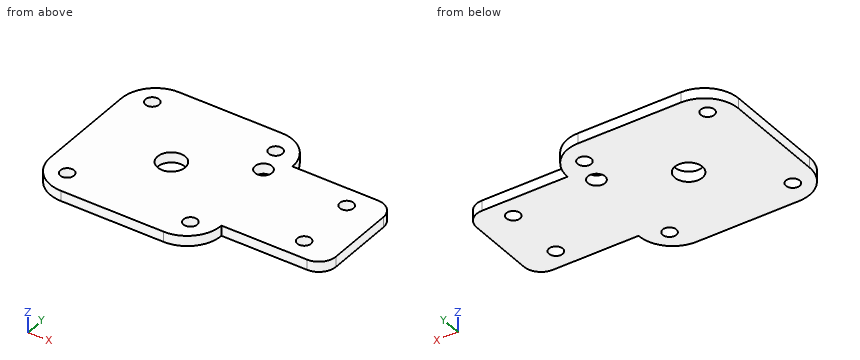
```python
from build123d import *

# Parameters (mm, degrees)
CROQUIS1_R              = 2.5
CROQUIS1_R_2            = 4.05
CROQUIS1_R_3            = 2
SALIENTE_EXTRUIR1_DEPTH = 3


with BuildPart() as part:
    # Croquis1 → Saliente-Extruir1 (new body)
    with BuildSketch(Plane.XY):
        with BuildLine():
            ThreePointArc((0, 40), (2.928932188, 47.071067812), (10, 50))
            Line((10, 50), (40, 50))
            ThreePointArc((40, 50), (47.071067812, 47.071067812), (50, 40))
            Line((50, 40), (50, 10))
            ThreePointArc((50, 10), (47.071067812, 2.928932188), (40, 0))
            Line((40, 0), (10, 0))
            ThreePointArc((10, 0), (2.928932188, 2.928932188), (0, 10))
            Line((0, 10), (0, 40))
        make_face()
        with Locations((45, 35)):
            Circle(CROQUIS1_R, mode=Mode.SUBTRACT)
        with Locations((25, 25)):
            Circle(CROQUIS1_R_2, mode=Mode.SUBTRACT)
        with Locations((43, 43)):
            Circle(CROQUIS1_R_3, mode=Mode.SUBTRACT)
        with Locations((7, 43)):
            Circle(CROQUIS1_R_3, mode=Mode.SUBTRACT)
        with Locations((43, 7)):
            Circle(CROQUIS1_R_3, mode=Mode.SUBTRACT)
        with Locations((7, 7)):
            Circle(CROQUIS1_R_3, mode=Mode.SUBTRACT)
        with BuildLine():
            ThreePointArc((75, 40), (78.535533906, 38.535533906), (80, 35))
            Line((80, 35), (80, 15))
            ThreePointArc((80, 15), (78.535533906, 11.464466094), (75, 10))
            Line((75, 10), (50, 10))
            Line((50, 10), (50, 40))
            Line((50, 40), (75, 40))
        make_face()
        with Locations((70, 16)):
            Circle(CROQUIS1_R_3, mode=Mode.SUBTRACT)
        with Locations((70, 34)):
            Circle(CROQUIS1_R_3, mode=Mode.SUBTRACT)
    extrude(amount=SALIENTE_EXTRUIR1_DEPTH)


solid = part.part
```
Check sheet for the modelled part. Datum: model origin and axes. Units: mm. Round coordinates to 2 decimals unless told otherwise and drop trailing zeros. Order: outer loops, then holes, each group sorted by start corner. A loop starts at its lowest first (then second) coordinate and runs counter-clockwise, first axis right, second up. Notation, with made-up numbers: M 34.5,-18 L 88.5,-18 A30 cw 88.5,9 Z; hole C 84.25,5.25 d8. An arc over 180 degrees is marked long. Answer in a Markdown table with one row per item.
(1) Section check A-A on x = 25. Record the boundary of the cut face in (y, z).
Findings:
| item | result |
|---|---|
| outline | M 0,0 L 20.95,0 L 20.95,3 L 0,3 Z; M 29.05,0 L 50,0 L 50,3 L 29.05,3 Z |
(2) Material ranges on line 1 along Y through (x, z) = (43, 2.35); line 2 along Y through (x, z) = (52.5, 2.55); line 3 along Y through (x, z) = (7, 1.85), recorded low to high. Write a range as from..to.
Findings:
| item | result |
|---|---|
| line 1 | y = 0.46..5, 9..33.5, 36.5..41, 45..49.54 |
| line 2 | y = 10..40 |
| line 3 | y = 0.46..5, 9..41, 45..49.54 |
(3) Gauge pin test, flat ends, axial feed: pin 1 (2.5 mm diameter, centred on x = 70, y = 16, fed in from -Z); pin 2 (0.9 mm diameter, centred on x = 58.5, z = 1.5, fed in from -Y). Record the tip position at first contact, or that the pin passes through.
Findings:
| item | result |
|---|---|
| pin 1 | passes through |
| pin 2 | stops at y = 10 |
(4) Section check C-C on y = 43. Record the boundary of the cut face in (x, z).
Findings:
| item | result |
|---|---|
| outline | M 0.46,0 L 5,0 L 5,3 L 0.46,3 Z; M 9,0 L 41,0 L 41,3 L 9,3 Z; M 45,0 L 49.54,0 L 49.54,3 L 45,3 Z |
(5) Section check D-D on x = 70. Record the boundary of the cut face in (y, z).
Findings:
| item | result |
|---|---|
| outline | M 10,0 L 14,0 L 14,3 L 10,3 Z; M 18,0 L 32,0 L 32,3 L 18,3 Z; M 36,0 L 40,0 L 40,3 L 36,3 Z |
(6) Section check B-B on z = 1.6. Give the number of separate pieces and of enclosed holes in the cut face, plus the area to 3 significant figures.
Findings:
| item | result |
|---|---|
| separate pieces | 1 |
| enclosed holes | 8 |
| area | 3,160 mm^2 |
